from build123d import *

# Parameters (mm, degrees)
SKETCH1_W               = 20
SKETCH1_H               = 18
BOSS_EXTRUDE1_DEPTH     = 6
SKETCH2_W               = 20
SKETCH2_H               = 3
BOSS_EXTRUDE2_DEPTH     = 3
SKETCH3_R               = 2.125
CUT_EXTRUDE1_DEPTH      = 1
CUT_EXTRUDE1_DEPTH_BACK = 10
CHAMFER1_SIZE           = 3
CHAMFER2_SIZE           = 5
CHAMFER3_SIZE           = 1.5


with BuildPart() as part:
    # Sketch1 → Boss-Extrude1 (new body)
    with BuildSketch(Plane(origin=(0, 0, 0), x_dir=(1, 0, 0), z_dir=(0, 1, 0))):
        Rectangle(SKETCH1_W, SKETCH1_H)
    extrude(amount=BOSS_EXTRUDE1_DEPTH)

    # Sketch2 → Boss-Extrude2 (add)
    with BuildSketch(Plane(origin=(0, 6, 0), x_dir=(1, 0, 0), z_dir=(0, 1, 0))):
        with Locations((0, 7.5)):
            Rectangle(SKETCH2_W, SKETCH2_H)
    extrude(amount=BOSS_EXTRUDE2_DEPTH)

    # Sketch3 → Cut-Extrude1 (cut, two sides)
    with BuildSketch(Plane.XZ) as cut_extrude1_sk:
        with Locations((0, 1.5)):
            Circle(SKETCH3_R)
    extrude(amount=CUT_EXTRUDE1_DEPTH, mode=Mode.SUBTRACT)
    extrude(cut_extrude1_sk.sketch, amount=-CUT_EXTRUDE1_DEPTH_BACK, mode=Mode.SUBTRACT)

    # Chamfer1
    chamfer1_edges = [part.edges().sort_by_distance(p)[0] for p in [
        (10, 0, 0),
        (0, 0, 9),
        (-10, 0, 0),
    ]]
    chamfer(chamfer1_edges, length=CHAMFER1_SIZE)

    # Chamfer2
    chamfer2_edges = [part.edges().sort_by_distance(p)[0] for p in [
        (0, 0, -9),
    ]]
    chamfer(chamfer2_edges, length=CHAMFER2_SIZE)

    # Chamfer3
    chamfer3_edges = [part.edges().sort_by_distance(p)[0] for p in [
        (0, 9, -9),
        (-10, 7, -9),
        (10, 7, -9),
    ]]
    chamfer(chamfer3_edges, length=CHAMFER3_SIZE)


solid = part.part
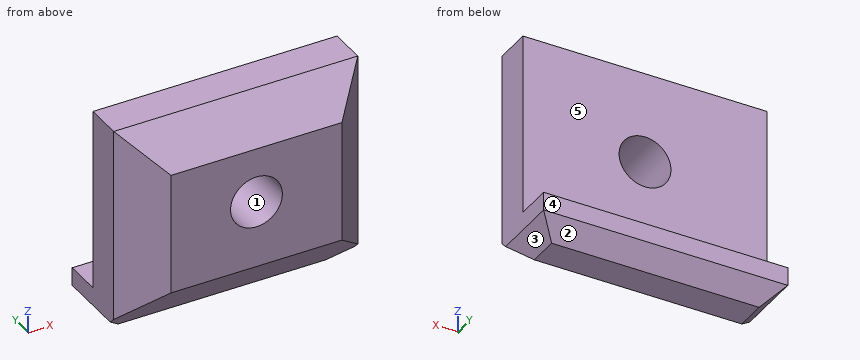
Can you work these out from the model? Positions are in its coordinate system, mm. Face numbers are marked on the shaded views. A direction names the side the tool comes from. Coordinates: 2 decimals unless noted, no trailing zeros. Write each loop counter-clockwise with the first axis right and the second up, starting at its lowest first coordinate (ties: lowest second). Pieces come first, ordered by that corner, then holes. Notation, with made-up numbers: (1.25, 37) - (6.25, 37) arc R20 cw to (6.25, 44) - close; hole circle Ø11 at (62, 11.5). An arc over 180 degrees is marked (long way). Return JSON: item names as keys, results as strings. Group by question number.
Item 1: If we section it at D-D (y = 7.25): Write out the boundary of the cut face in (x, z), then the cut area to 4 significant figures.
Item 2: If we section it at B-B (z = 1.5): Write out the boundary of the cut face in (x, y) (3 decimals).
Item 3: If we section it at A-A (x = 0): Write out the boundary of the cut face in (y, z) (3 decimals).
Item 4: If we section it at C-C (y = 2.25): Write out the boundary of the cut face in (x, z) (3 decimals).
Item 5: I'm going to push flat-ended pins straight in: pin 1 Ø0.9 at (x, y) = (2, 8) entering from +Z; pin 2 Ø7.5 at (x, z) = (-2, 1) entering from +Y; pin 3 Ø2.5 at (x, z) = (0, 1.5) entering from +Y. Where does each tip first touch, or does it pass through?
Item 6: We'd pull the mould along X, two halves only. Please class the marked faces 1, 2 and 3: pulls with the +X half, pulls with the -X half, needs draft (parallel to the pull), parting line crosses it, or undercut.
Item 7: Please list where these lines run through material, in increasing order: probe 1 along Z at (x, y) = (7.5, 6.5); probe 2 along Z at (x, y) = (-4.5, 3.5); probe 3 along Y at (x, z) = (2.5, 2.25).
Item 8: Which directions (+Z, -Z, +X, -X, +Y, -Y) give clear straight access to the entire face, cutting with the end or side of a thin tool? Please do the marked faces 4 and 5.
Return value:
{
 "1": {"outline": "(-10, -7.5) - (-8.5, -9) - (8.5, -9) - (10, -7.5) - (10, -6) - (-10, -6) - close", "area": "57.75 mm^2"},
 "2": {"outline": "(-10, 3) - (-7, 0) - (-2.125, 0) - (-2.125, 6) - (-10, 6) - close; (2.125, 0) - (7, 0) - (10, 3) - (10, 6) - (2.125, 6) - close"},
 "3": {"outline": "(0, -4) - (5, -9) - (7.5, -9) - (9, -7.5) - (9, -6) - (6, -6) - (6, -0.625) - (0, -0.625) - close; (0, 3.625) - (6, 3.625) - (6, 9) - (3, 9) - (0, 6) - close"},
 "4": {"outline": "(-9.25, -6.25) - (9.25, -6.25) - (9.25, 8.25) - (-9.25, 8.25) - close; hole circle Ø4.25 at (0, 1.5)"},
 "5": {"pin 1": "stops at z = -6", "pin 2": "stops at y = 6", "pin 3": "passes through"},
 "6": {"face 1": "undercut", "face 2": "needs draft", "face 3": "pulls with the +X half"},
 "7": {"probe 1": "z = -9 to -6", "probe 2": "z = -7.5 to 9", "probe 3": "y = 0 to 6"},
 "8": {"face 4": "+Z, -Z, +X, -X, +Y", "face 5": "+Z, +X, -X, +Y"}
}
